Here's how the part is built. I have some questions about the finished solid (model axes, mm). A direction names the side the tool comes from. Round coordinates to 2 decimals unless told otherwise and drop trailing zeros. Loops run counter-clockwise (first coordinate to the right, second up) from the corner with the lowest first, then second, coordinate; pieces in that order, holes last. Notation, with made-up numbers: M 39.25,-18.5 L 51.25,-18.5 A27 ccw 51.25,11.5 Z; hole C -29.5,-25 d11. An arc over 180 degrees is marked long. Use a Markdown table: item, result.
```python
from build123d import *

# Parameters (mm, degrees)
F1_DEPTH = 22
F2_W     = 2
F2_H     = 2.5
F2_W_2   = 3
F4_DEPTH = 15
F6_W     = 3
F6_H     = 3


with BuildPart() as f1:
    # F0 (on Front) → F1 (new body)
    with BuildSketch(Plane.XZ):
        Polygon((-22.3971781656, 0), (-28.3971781656, 0), (-28.3971781656, -2), (-20.3971781656, -2), (-20.3971781656, 5), (13.6028218344, 5), (15.6028218344, 5), (15.6028218344, 0), (9.6028218344, 0), (9.6028218344, -2), (18.6028218344, -2), (18.6028218344, 7), (-22.3971781656, 7), align=None)
    extrude(amount=F1_DEPTH)

    # F2 (on face) → F4 (cut)
    with BuildSketch(Plane.XZ.offset(22)):
        Polygon((-20.3971781656, 0), (-22.3971781656, 0), (-28.3971781656, 0), (-28.3971781656, -2), (-20.3971781656, -2), align=None)
        Polygon((18.6028218344, -2), (18.6028218344, 0), (15.6028218344, 0), (9.6028218344, 0), (9.6028218344, -2), align=None)
        with Locations((-21.3971781656, 1.25)):
            Rectangle(F2_W, F2_H)
        with Locations((17.1028218344, 1.25)):
            Rectangle(F2_W_2, F2_H)
    extrude(amount=-F4_DEPTH, mode=Mode.SUBTRACT)

    # F7: sweep along a path in F3
    with BuildLine(Plane.YZ) as f7_path:
        Line((-22.250123322, 8.247365728), (-5, 8.247365728))
        ThreePointArc((-5, 8.247365728), (-1.4644660941, 9.7118318221), (0, 13.247365728))
        Line((0, 13.247365728), (0, 33.247365728))
        ThreePointArc((0, 33.247365728), (-1.4644660941, 36.782899634), (-5, 38.247365728))
        Line((-5, 38.247365728), (-22.250123322, 38.247365728))
    # F6 (on offset) → F7 (sweep)
    with BuildSketch(Plane.XZ.offset(22)):
        with Locations((0, 8.247365728)):
            Rectangle(F6_W, F6_H)
    sweep(path=f7_path.line)

    # F8: F1 across plane


with BuildPart() as f1_1:
    add(f1.part)
    add(f1.part.mirror(Plane.XZ.offset(22)))


solid = f1_1.part
```
Q1. For faces 5 (the flat face through (-25, -41, 0)), 6 (the flat face through (0, -1.5, 23)), 7 (the flat face through (9.603, -41, -1)), 8 (the flat face through (-24, -7, -1)), which set-ups out of +Z, -Z, +X, -X, +Y, -Y let a thin tool reach every point of the face, with its end or its side?
Return value:
| item | result |
|---|---|
| face 5 | +Z, -X, +Y, -Y |
| face 6 | +X, -X |
| face 7 | -Z, +Y, -Y |
| face 8 | -Z, +X, -X |
Q2. I need wall thicknesses on line 1 (Z direction, x = 1, y = -11.5); line 2 (Z direction, x = 11, y = -1.5); line 3 (Y direction, x = -1, z = 18.5). Which ranges of each line are inside material? Lowest first, please. Write a range as from..to.
Return value:
| item | result |
|---|---|
| line 1 | z = 5..9.75, 36.75..39.75 |
| line 2 | z = -2..0, 5..7 |
| line 3 | y = -45.5..-42.5, -1.5..1.5 |
Q3. Imagine slicing it at D-D, the plane y = -6. Please give me the cut outline in (x, z), then the cut area to 3 significant figures.
Return value:
| item | result |
|---|---|
| outline | M -28.4,-2 L -20.4,-2 L -20.4,5 L 15.6,5 L 15.6,0 L 9.6,0 L 9.6,-2 L 18.6,-2 L 18.6,7 L 1.5,7 L 1.5,9.75 L -1.5,9.75 L -1.5,7 L -22.4,7 L -22.4,0 L -28.4,0 Z; M -1.5,36.75 L 1.5,36.75 L 1.5,39.75 L -1.5,39.75 Z |
| area | 158 mm^2 |
Q4. Imagine slicing it at C-C, the plane z = 30.5. Please give me the cut outline in (x, y).
Return value:
| item | result |
|---|---|
| outline | M -1.5,-45.5 L 1.5,-45.5 L 1.5,-42.5 L -1.5,-42.5 Z; M -1.5,-1.5 L 1.5,-1.5 L 1.5,1.5 L -1.5,1.5 Z |
Q5. We'd pull the mould along Z, two halves only. Please class faces 1 (the flat face through (-28.397, -3, -1)), 2 (the flat face through (15.603, -22, 3)), 3 (the flat face through (0, -42.5, 23)), 4 (the flat face through (-24, -3, -2)): pulls with the +Z half, pulls with the -Z half, needs draft (parallel to the pull), parting line crosses it, or undercut.
Return value:
| item | result |
|---|---|
| face 1 | needs draft |
| face 2 | undercut |
| face 3 | undercut |
| face 4 | pulls with the -Z half |
Q6. Will these pins go through, and if not, where does the flat tip stop? P1, Ø2, axis at x = -25.5, z = -0.5, coming from the -Y side; P2, Ø20.5, axis at x = -7.5, y = -16.5, coming from the +Z side; P3, Ø10, axis at y = -32.5, z = 14.5, coming from the +X side; P4, Ø3.5, axis at x = 0, y = -25.5, coming from the -Z side.
Return value:
| item | result |
|---|---|
| P1 | stops at y = -44 |
| P2 | stops at z = 39.75 |
| P3 | stops at x = 1.5 |
| P4 | stops at z = 5 |
Q7. Imagine slicing it at A-A, the plane z = 4. Please give me the cut outline in (x, y), then the cut area to 3 significant figures.
Return value:
| item | result |
|---|---|
| outline | M -22.4,-44 L -20.4,-44 L -20.4,0 L -22.4,0 Z; M 15.6,-44 L 18.6,-44 L 18.6,0 L 15.6,0 Z |
| area | 220 mm^2 |
Q8. Imagine slicing it at B-B, the plane y = -11.5. Please give me the cut outline in (x, z).
Return value:
| item | result |
|---|---|
| outline | M -22.4,2.5 L -20.4,2.5 L -20.4,5 L 15.6,5 L 15.6,2.5 L 18.6,2.5 L 18.6,7 L 1.5,7 L 1.5,9.75 L -1.5,9.75 L -1.5,7 L -22.4,7 Z; M -1.5,36.75 L 1.5,36.75 L 1.5,39.75 L -1.5,39.75 Z |
